from build123d import *

# Parameters (mm, degrees)
EXTRUDE_1_DEPTH      = 4.5
EXTRUDE_1_DEPTH_BACK = 4.5
EXTRUDE_2_DEPTH      = 3.175
EXTRUDE_2_DEPTH_BACK = 3.175
EXTRUDE_3_DEPTH      = 12.5
EXTRUDE_3_DEPTH_BACK = 12.5
SKETCH_4_R           = 1.5
EXTRUDE_4_DEPTH      = 25


with BuildPart() as part:
    # 草图1 → 凸台-拉伸1 (new, two sides: drawn at the far end of the back side and taken through both)
    with BuildSketch(Plane(origin=(11.5, 0, 0), x_dir=(0, 0, -1), z_dir=(1, 0, 0)).offset(-EXTRUDE_1_DEPTH_BACK)):
        with BuildLine():
            Line((-8, 16.7), (-8, 15.478695035))
            ThreePointArc((-8, 15.478695035), (-7.765507447, 15.055013793), (-7.281976818, 15.028732935))
            ThreePointArc((-7.281976818, 15.028732935), (-4.801971314, 15.994720113), (-2.2, 16.554455594))
            Line((-2.2, 16.554455594), (-2.2, 19.9))
            Line((-2.2, 19.9), (-1.5, 19.9))
            Line((-1.5, 19.9), (-1.5, 20.9))
            Line((-1.5, 20.9), (1.5, 20.9))
            Line((1.5, 20.9), (1.5, 19.9))
            Line((1.5, 19.9), (2.2, 19.9))
            Line((2.2, 19.9), (2.2, 16.554455594))
            ThreePointArc((2.2, 16.554455594), (4.801971275, 15.994720125), (7.281976744, 15.02873297))
            ThreePointArc((7.281976744, 15.02873297), (7.765507412, 15.055013771), (8, 15.478695035))
            Line((8, 15.478695035), (8, 16.7))
            Line((8, 16.7), (5, 20.9))
            Line((5, 20.9), (5, 27.9))
            Line((5, 27.9), (-5, 27.9))
            Line((-5, 27.9), (-5, 20.9))
            Line((-5, 20.9), (-8, 16.7))
        make_face()
    extrude(amount=EXTRUDE_1_DEPTH + EXTRUDE_1_DEPTH_BACK)

    # 草图2 → 凸台-拉伸2 (add, two sides: drawn at the far end of the back side and taken through both)
    with BuildSketch(Plane(origin=(11.5, 0, 0), x_dir=(0, 0, -1), z_dir=(1, 0, 0)).offset(-EXTRUDE_2_DEPTH_BACK)):
        with BuildLine():
            Line((17.197704205, 0.281016159), (17.128241699, 4.532001712))
            ThreePointArc((17.128241699, 4.532001712), (12.888690566, 14.42260896), (2.930137065, 18.5))
            Line((2.930137065, 18.5), (-2.930137065, 18.5))
            ThreePointArc((-2.930137065, 18.5), (-12.888690566, 14.42260896), (-17.128241699, 4.532001712))
            Line((-17.128241699, 4.532001712), (-17.197704205, 0.281016159))
            ThreePointArc((-17.197704205, 0.281016159), (0, -17.2), (17.197704205, 0.281016159))
        make_face()
        with BuildLine():
            Line((16.6, 0), (16.6, 4))
            ThreePointArc((16.6, 4), (12.440916293, 14.040916293), (2.4, 18.2))
            Line((2.4, 18.2), (-2.4, 18.2))
            ThreePointArc((-2.4, 18.2), (-12.440916293, 14.040916293), (-16.6, 4))
            Line((-16.6, 4), (-16.6, 0))
            ThreePointArc((-16.6, 0), (0, -16.6), (16.6, 0))
        make_face(mode=Mode.SUBTRACT)
    extrude(amount=EXTRUDE_2_DEPTH + EXTRUDE_2_DEPTH_BACK)

    # 草图3 → 凸台-拉伸3 (add, two sides: drawn at the far end of the back side and taken through both)
    with BuildSketch(Plane(origin=(11.5, 0, 0), x_dir=(0, 0, -1), z_dir=(1, 0, 0)).offset(-EXTRUDE_3_DEPTH_BACK)):
        Polygon((-2.2, 20.3), (-2.2, 16.6), (2.2, 16.6), (2.2, 20.3), (1.5, 20.3), (1.5, 21.3), (-1.5, 21.3), (-1.5, 20.3), align=None)
    extrude(amount=EXTRUDE_3_DEPTH + EXTRUDE_3_DEPTH_BACK)

    # 草图4 → 凸台-拉伸4 (add)
    with BuildSketch(Plane(origin=(11.5, 0, 0), x_dir=(0, 0, -1), z_dir=(1, 0, 0))):
        with Locations((0, 18.55)):
            Circle(SKETCH_4_R)
    extrude(amount=EXTRUDE_4_DEPTH)


solid = part.part
Verification items for the finished model (mm, model axes). A direction names the side the tool comes from. Round coordinates to 2 decimals unless told otherwise and drop trailing zeros. Loops run counter-clockwise (first coordinate to the right, second up) from the corner with the lowest first, then second, coordinate; pieces in that order, holes last. Notation, with made-up numbers: (51.25, 17.5) - (77.25, 17.5) arc R9 cw to (77.25, 26.5) - close; hole circle Ø3 at (-33.75, 42.5). An arc over 180 degrees is marked (long way). Use a Markdown table: item, result. Add a question column.
1. Section check A-A, the plane z = 0. Record the boundary of the cut face in (x, y) (3 decimals), plus the area to 3 significant figures.
2. Thickness scan on probe 1 along Z at (x, y) = (22, 19); probe 2 along Z at (x, y) = (12.5, 11); probe 3 along Y at (x, z) = (14.5, 1). Record the ranges inside material, lowest first. Write a range as [from, to].
3. Gauge pin test, flat ends, axial feed: pin 1 (17 mm diameter, centred on y = 1, z = -6.5, fed in from -X); pin 2 (4 mm diameter, centred on y = 20.5, z = 3, fed in from +X); pin 3 (1.8 mm diameter, centred on x = 1.5, y = 19, fed in from -Z); pin 4 (2 mm diameter, centred on x = 11, y = 13, fed in from -Z). Record the tip position at first contact, or that the pin passes through.
4. Section check D-D, the plane z = 6. Record the boundary of the cut face in (x, y) (3 decimals).
5. Section check C-C, the plane x = 4. Record the boundary of the cut face in (y, z), plus the area to 3 significant figures.
6. Release check for a two-part mould opening along Z. For faces 1 (the face through (11, 27.9, 0)), 2 (the face through (11, 2, 16.6)), 3 (the face through (20, 18, -2.2)) record: released by +Z, released by -Z, zero draft, split by the parting line, or undercut.
7. Section check B-B, the plane y = 11.5. Record the boundary of the cut face in (x, z) (3 decimals), plus the area to 3 significant figures.
8. Access from +Z, -Z, +X, -X, +Y, -Y to the whole of each face (thin tool, end or side, straight path). Record for faces 4 (the face through (20, 21.3, 0)), 5 (the face through (11, 16.6, 0)), 6 (the face through (20, 18, 2.2)), 7 (the face through (24, 20, 1)).
Checks:
| question | item | result |
|---|---|---|
| 1 | outline | (-1, 16.6) - (24, 16.6) - (24, 17.05) - (36.5, 17.05) - (36.5, 20.05) - (24, 20.05) - (24, 21.3) - (16, 21.3) - (16, 27.9) - (7, 27.9) - (7, 21.3) - (-1, 21.3) - close; (8.325, -17.2) - (14.675, -17.2) - (14.675, -16.6) - (8.325, -16.6) - close |
| 1 | area | 218 mm^2 |
| 2 | probe 1 | z = [-2.2, 2.2] |
| 2 | probe 2 | z = [-15.45, -14.75], [14.75, 15.45] |
| 2 | probe 3 | y = [-17.17, -16.57], [16.6, 27.9] |
| 3 | pin 1 | passes through |
| 3 | pin 2 | stops at x = 24 |
| 3 | pin 3 | stops at z = -2.2 |
| 3 | pin 4 | stops at z = -14.86 |
| 4 | outline | (7, 15.585) - (16, 15.585) - (16, 19.5) - (7, 19.5) - close; (8.325, -16.12) - (14.675, -16.12) - (14.675, -15.478) - (8.325, -15.478) - close |
| 5 | outline | (16.6, -2.2) - (20.3, -2.2) - (20.3, -1.5) - (21.3, -1.5) - (21.3, 1.5) - (20.3, 1.5) - (20.3, 2.2) - (16.6, 2.2) - close |
| 5 | area | 19.3 mm^2 |
| 6 | face 1 | zero draft |
| 6 | face 2 | undercut |
| 6 | face 3 | released by -Z |
| 7 | outline | (8.325, -15.169) - (14.675, -15.169) - (14.675, -14.458) - (8.325, -14.458) - close; (8.325, 14.458) - (14.675, 14.458) - (14.675, 15.169) - (8.325, 15.169) - close |
| 7 | area | 9.04 mm^2 |
| 8 | face 4 | +Z, -Z, +X, +Y |
| 8 | face 5 | +X, -X |
| 8 | face 6 | +Z, +X, +Y, -Y |
| 8 | face 7 | +X |
